```python
from build123d import *

# Parameters (mm, degrees)
CHAMFER_1_SIZE            = 1
HOLE_WIZARD_8_0_8_1_D     = 8
HOLE_WIZARD_8_0_8_1_DEPTH = 70
HOLE_WIZARD_8_0_8_1_TIP   = 2.403442476
CHAMFER_2_SIZE            = 5
M10X1_0_1_D               = 9
M10X1_0_1_DEPTH           = 15
M10X1_0_1_TIP             = 2.703872786
HOLE_WIZARD_6_0_6_4_D     = 6
HOLE_WIZARD_6_0_6_4_DEPTH = 35
HOLE_WIZARD_6_0_6_4_TIP   = 1.802581857
SKETCH_8_R                = 8.5
CUT_EXTRUDE_1_DEPTH       = 35


with BuildPart() as part:
    # 草图1 → 旋转1 (revolve)
    with BuildSketch(Plane.XY):
        Polygon((0, 0), (0, 42.5), (10, 42.5), (10, 35), (385, 35), (385, 0), align=None)
    revolve(axis=Axis((385, 0, 0), (-1, 0, 0)))

    # 倒角1
    chamfer_1_edges = [part.edges().sort_by_distance(p)[0] for p in [
        (10, -42.5, 0),
        (0, -42.5, 0),
    ]]
    chamfer(chamfer_1_edges, length=CHAMFER_1_SIZE)

    # Ø8.0 (8) 直径孔1
    with Locations(Plane(origin=(0, 0, 0), x_dir=(0, -1, 0), z_dir=(-1, 0, 0))):
        with Locations((0, 0)):
            Hole(HOLE_WIZARD_8_0_8_1_D / 2, depth=HOLE_WIZARD_8_0_8_1_DEPTH)
            with Locations((0, 0, -(HOLE_WIZARD_8_0_8_1_DEPTH + HOLE_WIZARD_8_0_8_1_TIP / 2))):  # 118° drill point
                Cone(0, HOLE_WIZARD_8_0_8_1_D / 2, HOLE_WIZARD_8_0_8_1_TIP, mode=Mode.SUBTRACT)

    # 倒角2
    chamfer_2_edges = [part.edges().sort_by_distance(p)[0] for p in [
        (385, -35, 0),
    ]]
    chamfer(chamfer_2_edges, length=CHAMFER_2_SIZE)

    # M10x1.0 螺纹孔1
    with Locations(Plane(origin=(0, 0, 0), x_dir=(0, -1, 0), z_dir=(-1, 0, 0))):
        with Locations((0, 0)):
            Hole(M10X1_0_1_D / 2, depth=M10X1_0_1_DEPTH)
            with Locations((0, 0, -(M10X1_0_1_DEPTH + M10X1_0_1_TIP / 2))):  # 118° drill point
                Cone(0, M10X1_0_1_D / 2, M10X1_0_1_TIP, mode=Mode.SUBTRACT)

    # Ø6.0 (6) 直径孔4
    with Locations(Plane(origin=(0, 35, 0), x_dir=(1, 0, 0), z_dir=(0, 1, 0))):
        with Locations((65, 0)):
            Hole(HOLE_WIZARD_6_0_6_4_D / 2, depth=HOLE_WIZARD_6_0_6_4_DEPTH)
            with Locations((0, 0, -(HOLE_WIZARD_6_0_6_4_DEPTH + HOLE_WIZARD_6_0_6_4_TIP / 2))):  # 118° drill point
                Cone(0, HOLE_WIZARD_6_0_6_4_D / 2, HOLE_WIZARD_6_0_6_4_TIP, mode=Mode.SUBTRACT)

    # 草图8 → 切除-拉伸1 (cut, symmetric)
    with BuildSketch(Plane(origin=(0, 0, 0), x_dir=(1, 0, 0), z_dir=(0, 1, 0))):
        with Locations((217.5, 0)):
            Circle(SKETCH_8_R)
    extrude(amount=CUT_EXTRUDE_1_DEPTH, both=True, mode=Mode.SUBTRACT)


solid = part.part
```
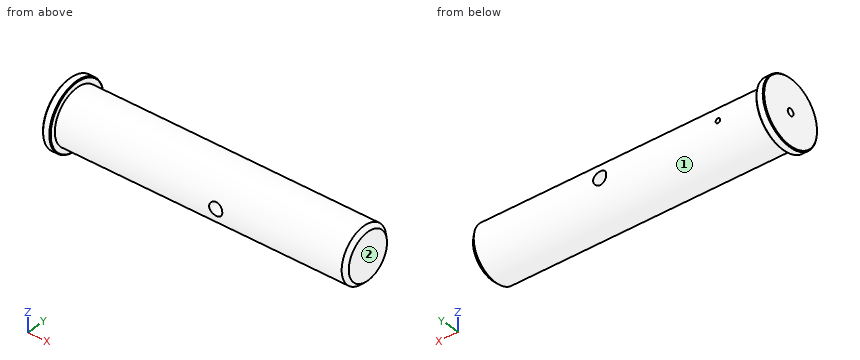
For this review, take the finished solid that the model builds, in its own axes (mm). Face numbers are marked on the shaded views. A direction names the side the tool comes from. Coordinates: 2 decimals unless noted, no trailing zeros. Loops run counter-clockwise (first coordinate to the right, second up) from the corner with the lowest first, then second, coordinate; pieces in that order, holes last. Notation, with made-up numbers: (3, 89.25) -> (26, 89.25) arc R19 cw to (26, 103.25) -> close; hole circle Ø5 at (25.5, 56.25). An arc over 180 degrees is marked (long way). Return JSON: item names as keys, results as strings. Group by question number.
(1) Consider section C-C, the plane y = 26. Count the separate pieces of the cut face and the enclosed holes in it, plus the area to 3 significant figures.
(2) Consider section A-A, the plane x = 32.5. Give the boundary of the cut face in (y, z).
(3) To check wall thickness, follow L1, parallel to X at y = 15, z = 0; L2, parallel to Z at x = 30, y = 0; L3, parallel to Y at x = 4, z = 0. State the ranges of each line that lie inside material, in increasing order.
(4) Consider section D-D, the plane x = 297. Give the boundary of the cut face in (y, z).
(5) For pin 1 Ø6 at (x, z) = (107, 28.5) entering from +Y; pin 2 Ø5 at (x, z) = (65, 0) entering from +Y; pin 3 Ø10 at (x, y) = (75, 21) entering from +Z, all flat-tipped, find the tip position at first contact; note any pin that passes through.
(6) Tool access review of the marked faces 1 and 2: name each direction out of +Z, -Z, +X, -X, +Y, -Y from which nothing blocks a thin tool from reaching the whole face with its end or side.
(7) Consider section B-B, the plane x = 217.5. Give the boundary of the cut face in (y, z), plus the area to 3 significant figures.
Results below:
{
 "1": {"separate pieces": "1", "enclosed holes": "2", "area": "17,900 mm2"},
 "2": {"outline": "circle Ø70 at (0, 0); hole circle Ø8 at (0, 0)"},
 "3": {"L1": "x = 0 to 62, 68 to 209, 226 to 385", "L2": "z = -35 to -4, 4 to 35", "L3": "y = -42.5 to -4.5, 4.5 to 42.5"},
 "4": {"outline": "circle Ø70 at (0, 0)"},
 "5": {"pin 1": "stops at y = 23.97", "pin 2": "stops at y = -3.12", "pin 3": "stops at z = 31.13"},
 "6": {"face 1": "+X", "face 2": "+Z, -Z, +X, +Y, -Y"},
 "7": {"outline": "(-33.95, -8.5) arc R35 ccw to (33.95, -8.5) -> close; (-33.95, 8.5) -> (33.95, 8.5) arc R35 ccw to start", "area": "2,670 mm2"}
}
